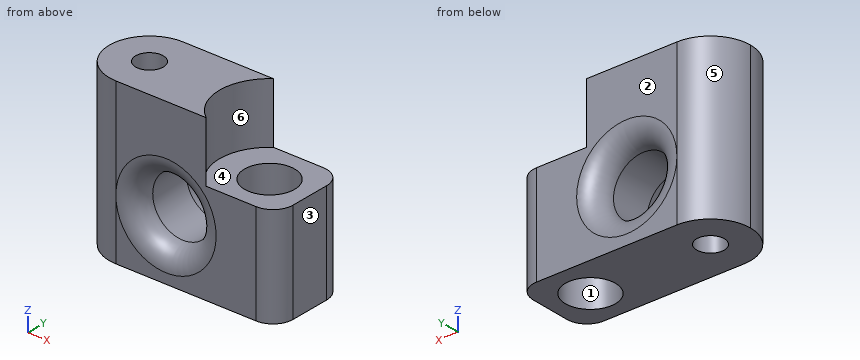
```python
from build123d import *

# Parameters (mm, degrees)
SKETCH2_W                   = 10.16
SKETCH2_H                   = 10.16
EXTRUDE2_DEPTH              = 20.32
FILLET1_R                   = 2.54
SKETCH5_W                   = 20.32
SKETCH5_H                   = 10.16
EXTRUDE3_DEPTH              = 15.24
FILLET3_R                   = 5.08
SKETCH9_R                   = 3.81
CUT_EXTRUDE1_DEPTH          = 35.077675977
FILLET4_R                   = 2.54
SKETCH10_R                  = 6.35
CUT_EXTRUDE2_DEPTH          = 7.62
F_1_4_0_25_DIAMETER_HOLE1_D = 6.35
F_6_32_TAPPED_HOLE1_D       = 3.5052


with BuildPart() as part:
    # Sketch2 → Extrude2 (new body)
    with BuildSketch(Plane.XY):
        with Locations((-5.08, 5.08)):
            Rectangle(SKETCH2_W, SKETCH2_H)
    extrude(amount=EXTRUDE2_DEPTH)

    # Fillet1
    fillet1_edges = [part.edges().sort_by_distance(p)[0] for p in [
        (0, 0, 10.16),
        (0, 10.16, 10.16),
    ]]
    fillet(fillet1_edges, radius=FILLET1_R)

    # Sketch5 → Extrude3 (add)
    with BuildSketch(Plane.ZY.offset(10.16)):
        with Locations((10.16, 5.08)):
            Rectangle(SKETCH5_W, SKETCH5_H)
    extrude(amount=EXTRUDE3_DEPTH)

    # Fillet3
    fillet3_edges = [part.edges().sort_by_distance(p)[0] for p in [
        (-25.4, 0, 10.16),
        (-25.4, 10.16, 10.16),
    ]]
    fillet(fillet3_edges, radius=FILLET3_R - 0.0001)  # a hair under: the kernel refuses the full size

    # Sketch9 → Cut-Extrude1 (cut, through all)
    with BuildSketch(Plane(origin=(0, 10.16, 0), x_dir=(-1, 0, 0), z_dir=(0, 1, 0))):
        with Locations((13.97, 7.62)):
            Circle(SKETCH9_R)
    extrude(amount=-CUT_EXTRUDE1_DEPTH, mode=Mode.SUBTRACT)

    # Fillet4
    fillet4_edges = [part.edges().sort_by_distance(p)[0] for p in [
        (-10.16, 0, 7.62),
        (-10.16, 10.16, 7.62),
    ]]
    fillet(fillet4_edges, radius=FILLET4_R)

    # Sketch10 → Cut-Extrude2 (cut)
    with BuildSketch(Plane.XY.offset(20.32)):
        with Locations((-5.08, 5.08)):
            Circle(SKETCH10_R)
    extrude(amount=-CUT_EXTRUDE2_DEPTH, mode=Mode.SUBTRACT)

    # 1/4 (0.25) Diameter Hole1 (through all)
    with Locations(Plane(origin=(-5.08, 5.047963929, 12.7), x_dir=(1, 0, 0), z_dir=(0, 0, 1))):
        with Locations((0, 0)):
            Hole(F_1_4_0_25_DIAMETER_HOLE1_D / 2)

    # #6-32 Tapped Hole1 (through all)
    with Locations(Plane(origin=(-20.32, 5.08, 20.32), x_dir=(1, 0, 0), z_dir=(0, 0, 1))):
        with Locations((0, 0)):
            Hole(F_6_32_TAPPED_HOLE1_D / 2)


solid = part.part
```
Here's how the part is built. I have some questions about the finished solid (model axes, mm). Face numbers are marked on the shaded views. A direction names the side the tool comes from. Give positions to 0.01 mm unless a question says otherwise; leave off trailing zeros. Order: outer loops, then holes, each group sorted by start corner. A loop starts at its lowest first (then second) coordinate and runs counter-clockwise, first axis right, second up. Notation, with made-up numbers: (46.25, 69) - (91.25, 69) arc R15 ccw to (91.25, 78) - close; hole circle Ø1 at (23, 36). An arc over 180 degrees is marked (long way). Answer as a JSON object with one key per item and string values. Group by question number.
Item 1: If we mould it in two halves opening along Y, with no side actions, what happens to the marked faces 1, 2, 3 and 4? For each: pulls with the +Y half, pulls with the -Y half, needs draft (parallel to the pull), parting line crosses it, or undercut.
Item 2: For P1, Ø5, axis at x = -22, z = 4, coming from the +Y side; P2, Ø3, axis at x = -4, y = 4, coming from the +Z side; P3, Ø9, axis at x = -13.97, z = 7.62, coming from the -Y side, each with a flat end and sliding along its axis, tell me the tip position at first contact or that it passes through.
Item 3: Please list where these lines run through material, in increasing order: probe 1 along Z at (x, y) = (-13.97, 6.2); probe 2 along Y at (x, z) = (-20.32, 8.75); probe 3 along Y at (x, z) = (-5.08, 8.5).
Item 4: If we section it at B-B on y = 4: Please give me the cut outline in (x, z), and give its area (3 significant figures).
Item 5: If we section it at D-D on z = 7.62: Give the number of separate pieces and of enclosed holes in the cut face, and give its area (3 significant figures).
Item 6: Which directions (+Z, -Z, +X, -X, +Y, -Y) give clear straight access to the entire face, cutting with the end or side of a thin tool? Please do the marked faces 5 and 6.
Item 7: If we section it at A-A on x = -13.97: Please give me the cut outline in (y, z), and give its area (3 significant figures).
Result set:
{
 "1": {"face 1": "undercut", "face 2": "pulls with the +Y half", "face 3": "needs draft", "face 4": "undercut"},
 "2": {"P1": "y = 10.16", "P2": "through", "P3": "y = 0.8"},
 "3": {"probe 1": "0 to 3.81, 11.43 to 20.32", "probe 2": "0 to 3.33, 6.83 to 10.16", "probe 3": "0 to 1.87, 8.22 to 10.16"},
 "4": {"outline": "(-25.28, 0) - (-21.7, 0) - (-21.7, 20.32) - (-25.28, 20.32) - close; (-18.94, 0) - (-8.08, 0) - (-8.08, 12.7) - (-11.34, 12.7) - (-11.34, 20.32) - (-18.94, 20.32) - close; (-2.08, 0) - (0, 0) - (0, 12.7) - (-2.08, 12.7) - close; hole circle Ø7.62 at (-13.97, 7.62)", "area": "250 mm²"},
 "5": {"separate pieces": "2", "enclosed holes": "2", "area": "120 mm²"},
 "6": {"face 5": "+Z, -Z, -X, +Y", "face 6": "+Z, +X"},
 "7": {"outline": "(0, 0) - (10.16, 0) - (10.16, 1.27) arc R2.54 ccw to (7.62, 3.81) - (2.54, 3.81) arc R2.54 ccw to (0, 1.27) - close; (0, 13.97) arc R2.54 ccw to (2.54, 11.43) - (7.62, 11.43) arc R2.54 ccw to (10.16, 13.97) - (10.16, 20.32) - (0, 20.32) - close", "area": "123 mm²"}
}
